```python
from build123d import *

# Parameters (mm, degrees)
F0_R     = 40
F0_R_2   = 25
F1_DEPTH = 30
F0_R_3   = 8
F2_DEPTH = 30
F3_SIZE  = 15


with BuildPart() as f1:
    # F0 (on Front) → F1 (new body)
    with BuildSketch(Plane.XZ):
        Circle(F0_R)
        Circle(F0_R_2, mode=Mode.SUBTRACT)
    extrude(amount=F1_DEPTH)

    # F0 (on Front) → F2 (join)
    with BuildSketch(Plane.XZ):
        Circle(F0_R)
        Circle(F0_R_2, mode=Mode.SUBTRACT)
        Circle(F0_R_2)
        Circle(F0_R_3, mode=Mode.SUBTRACT)
    extrude(amount=F2_DEPTH)

    # F3
    f3_edges = [f1.edges().sort_by_distance(p)[0] for p in [
        (-40, 0, 0),
    ]]
    chamfer(f3_edges, length=F3_SIZE)


solid = f1.part
```
Can you work these out from the model? Positions are in its coordinate system, mm. Coordinates: 2 decimals unless noted, no trailing zeros. Loops run counter-clockwise (first coordinate to the right, second up) from the corner with the lowest first, then second, coordinate; pieces in that order, holes last. Notation, with made-up numbers: (-23.5, 50) -> (34.5, 50) arc R10 cw to (34.5, 62) -> close; hole circle Ø8 at (39.5, 78.5). An arc over 180 degrees is marked (long way). Answer as a JSON object with one key per item and string values.
1) Imagine slicing it at C-C (y = -1.75). Please give me the cut outline in (x, z), then the cut area to 3 significant figures.
Results:
{"outline": "circle Ø53.5 at (0, 0); hole circle Ø16 at (0, 0)", "area": "2,050 mm^2"}
2) Imagine slicing it at B-B (z = 0). Please give me the cut outline in (x, y).
Results:
{"outline": "(-40, -30) -> (-8, -30) -> (-8, 0) -> (-25, 0) -> (-40, -15) -> close; (8, -30) -> (40, -30) -> (40, -15) -> (25, 0) -> (8, 0) -> close"}
3) Imagine slicing it at A-A (x = 0). Please give me the cut outline in (y, z), then the cut area to 4 significant figures.
Results:
{"outline": "(-30, -40) -> (-15, -40) -> (0, -25) -> (0, -8) -> (-30, -8) -> close; (-30, 8) -> (0, 8) -> (0, 25) -> (-15, 40) -> (-30, 40) -> close", "area": "1,695 mm^2"}
4) Thinking about a two-plate mould opening in X: for faces 1 (the face through (-1.73, -14.79, -7.81)), 2 (the face through (-8.67, -22.4, -39.05)), 3 (the face through (8.3, -30, 0.6)), which applies, pulls with the +X half, pulls with the -X half, needs draft (parallel to the pull), parting line crosses it, or undercut?
Results:
{"face 1": "undercut", "face 2": "parting line crosses it", "face 3": "needs draft"}
5) Imagine slicing it at D-D (y = -26.25). Please give me the cut outline in (x, z), then the cut area to 3 significant figures.
Results:
{"outline": "circle Ø80 at (0, 0); hole circle Ø16 at (0, 0)", "area": "4,830 mm^2"}
6) For P1, Ø10, axis at x = 27, y = -6, coming from the +Z side; P2, Ø1.5, axis at x = 31, z = -29, coming from the +Y side; P3, Ø5, axis at y = -8, z = 9, coming from the +X side; P4, Ø12, axis at y = -22, z = 5.5, coming from the -X side, each with a flat end and sliding along its axis, tell me the tip position at first contact or that it passes through.
Results:
{"P1": "stops at z = 25.48", "P2": "passes through", "P3": "stops at x = 34.42", "P4": "stops at x = -40"}
7) If I drill on line 1 (Z direction, x = 0, y = -21.75); line 2 (X direction, y = -23.25, z = -1); line 3 (Z direction, x = -1.5, y = -8.5), over which ranges is the centre line in solid material (lowest first)?
Results:
{"line 1": "z = -40 to -8, 8 to 40", "line 2": "x = -39.99 to -7.94, 7.94 to 39.99", "line 3": "z = -33.47 to -7.86, 7.86 to 33.47"}
